Could you check a few things on this model? Use its own coordinates, in mm. A direction names the side the tool comes from. Give positions to 0.01 mm unless a question says otherwise; leave off trailing zeros. Write each loop counter-clockwise with the first axis right and the second up, starting at its lowest first coordinate (ties: lowest second). Pieces come first, ordered by that corner, then holes. Notation, with made-up numbers: M 55.5,35 L 105.5,35 A19 cw 105.5,48 Z; hole C 20.25,39.5 d3. An arc over 180 degrees is marked long. Use one line per item in the form item = value.
from build123d import *

# Parameters (mm, degrees)
F0_R     = 2
F0_R_2   = 6
F0_W     = 51.13
F0_H     = 19.04
F1_DEPTH = 25


# Not quite as in the source:
# - ends of sketch curves that miss each other by under 0.0002 mm in the source are joined


with BuildPart() as f1:
    # F0 (on Front) → F1 (new body)
    with BuildSketch(Plane.XZ):
        with BuildLine():
            Line((-0.0546134975, 0), (0, 0))
            Line((0, 0), (39.9453865025, 1.14717e-05))
            Line((39.9453865025, 1.14717e-05), (39.9453865025, 10.0000114717))
            Line((39.9453865025, 10.0000114717), (29.9453865025, 10.0000114717))
            Line((29.9453865025, 10.0000114717), (29.9576031817, 39.0801515195))
            ThreePointArc((29.9576031817, 39.0801515195), (24.9768942877, 34.5421678148), (20, 39.0843347471))
            ThreePointArc((20, 39.0843347471), (19.9842488656, 39.3130102593), (19.9789948068, 39.5421673735))
            ThreePointArc((19.9789948068, 39.5421673735), (14.7708428858, 35.0052540588), (10, 40))
            ThreePointArc((10, 40), (5, 35), (0, 40))
            ThreePointArc((0, 40), (-5, 35), (-10, 40))
            ThreePointArc((-10, 40), (-15, 35), (-20, 40))
            ThreePointArc((-20, 40), (-25, 35), (-30, 40))
            Line((-30, 40), (-30, 10))
            Line((-30, 10), (-40, 10))
            Line((-40, 10), (-40, 0))
            Line((-40, 0), (-0.0546134975, 0))
        make_face()
        with Locations((-35, 5)):
            Circle(F0_R, mode=Mode.SUBTRACT)
        with Locations((34.9453865025, 5.0000114717)):
            Circle(F0_R, mode=Mode.SUBTRACT)
        with BuildLine():
            ThreePointArc((20, 39.0843347471), (24.9768942877, 34.5421678148), (29.9576031817, 39.0801515195))
            Line((29.9576031817, 39.0801515195), (29.9579896136, 40))
            Line((29.9579896136, 40), (29.9747937682, 80))
            ThreePointArc((29.9747937682, 80), (24.9873968841, 75.3547848935), (20, 80))
            Line((20, 80), (20, 40))
            Line((20, 40), (20, 39.0843347471))
        make_face()
        with BuildLine():
            Line((29.9579896136, 40), (29.9576031817, 39.0801515195))
            ThreePointArc((29.9576031817, 39.0801515195), (29.9789943656, 39.5400668544), (29.9579896136, 40))
        make_face()
        with BuildLine():
            Line((-30, 80), (-30, 40))
            ThreePointArc((-30, 40), (-25, 35), (-20, 40))
            Line((-20, 40), (-20, 80))
            ThreePointArc((-20, 80), (-25, 75), (-30, 80))
        make_face()
        with BuildLine():
            Line((-30, 120), (-30, 80))
            ThreePointArc((-30, 80), (-25, 75), (-20, 80))
            Line((-20, 80), (-20, 120))
            ThreePointArc((-20, 120), (-25, 115), (-30, 120))
        make_face()
        with BuildLine():
            ThreePointArc((20, 80), (24.9873968841, 75.3547848935), (29.9747937682, 80))
            Line((29.9747937682, 80), (29.9915979227, 120))
            ThreePointArc((29.9915979227, 120), (24.9957989614, 115.2049212963), (20, 120))
            Line((20, 120), (20, 80))
        make_face()
        with BuildLine():
            Line((-30, 140), (-30, 120))
            ThreePointArc((-30, 120), (-25, 115), (-20, 120))
            Line((-20, 120), (-20, 140))
            Line((-20, 140), (-30, 140))
        make_face()
        with BuildLine():
            ThreePointArc((20, 120), (24.9957989614, 115.2049212963), (29.9915979227, 120))
            Line((29.9915979227, 120), (30, 140))
            Line((30, 140), (20, 140))
            Line((20, 140), (20, 120))
        make_face()
        Polygon((-40, 140), (-30, 140), (-20, 140), (-10, 140), (0, 140), (10, 140), (20, 140), (30, 140), (40, 140), (40, 220), (30, 220), (-30, 220), (-40, 220), align=None)
        with Locations((-35, 215)):
            Circle(F0_R, mode=Mode.SUBTRACT)
        with Locations((-20, 156)):
            Circle(F0_R_2, mode=Mode.SUBTRACT)
        with Locations((-15, 170)):
            Circle(F0_R, mode=Mode.SUBTRACT)
        with Locations((-5, 156)):
            Circle(F0_R, mode=Mode.SUBTRACT)
        with Locations((-5, 170)):
            Circle(F0_R, mode=Mode.SUBTRACT)
        with Locations((5, 170)):
            Circle(F0_R, mode=Mode.SUBTRACT)
        with Locations((15, 170)):
            Circle(F0_R, mode=Mode.SUBTRACT)
        with Locations((0, 189.52)):
            Rectangle(F0_W, F0_H, mode=Mode.SUBTRACT)
        with Locations((35, 215)):
            Circle(F0_R, mode=Mode.SUBTRACT)
        Polygon((-30, 230), (-30, 220), (30, 220), (30, 230), (0, 230), align=None)
        Polygon((-20, 250), (-30, 230), (0, 230), (30, 230), (20, 250), (0, 250), align=None)
        Polygon((0, 300), (-20, 250), (0, 250), (20, 250), align=None)
        with BuildLine():
            Line((-20, 120), (-20, 80))
            ThreePointArc((-20, 80), (-15, 75), (-10, 80))
            Line((-10, 80), (-10, 120))
            ThreePointArc((-10, 120), (-15, 115), (-20, 120))
        make_face()
        with BuildLine():
            Line((-10, 120), (-10, 80))
            ThreePointArc((-10, 80), (-5, 75), (0, 80))
            Line((0, 80), (0, 120))
            ThreePointArc((0, 120), (-5, 115), (-10, 120))
        make_face()
        with BuildLine():
            ThreePointArc((0, 80), (5, 75), (10, 80))
            Line((10, 80), (10, 120))
            ThreePointArc((10, 120), (5, 115), (0, 120))
            Line((0, 120), (0, 80))
        make_face()
        with BuildLine():
            ThreePointArc((10, 80), (15, 75), (20, 80))
            Line((20, 80), (20, 120))
            ThreePointArc((20, 120), (15, 115), (10, 120))
            Line((10, 120), (10, 80))
        make_face()
        with BuildLine():
            ThreePointArc((19.9789948068, 39.5421673735), (19.9842488656, 39.7713244878), (20, 40))
            Line((20, 40), (20, 80))
            ThreePointArc((20, 80), (15, 75), (10, 80))
            Line((10, 80), (10, 40))
            ThreePointArc((10, 40), (14.7708428858, 35.0052540588), (19.9789948068, 39.5421673735))
        make_face()
        with BuildLine():
            ThreePointArc((0, 40), (5, 35), (10, 40))
            Line((10, 40), (10, 80))
            ThreePointArc((10, 80), (5, 75), (0, 80))
            Line((0, 80), (0, 40))
        make_face()
        with BuildLine():
            Line((-10, 80), (-10, 40))
            ThreePointArc((-10, 40), (-5, 35), (0, 40))
            Line((0, 40), (0, 80))
            ThreePointArc((0, 80), (-5, 75), (-10, 80))
        make_face()
        with BuildLine():
            Line((-20, 80), (-20, 40))
            ThreePointArc((-20, 40), (-15, 35), (-10, 40))
            Line((-10, 40), (-10, 80))
            ThreePointArc((-10, 80), (-15, 75), (-20, 80))
        make_face()
        with BuildLine():
            Line((-20, 140), (-20, 120))
            ThreePointArc((-20, 120), (-15, 115), (-10, 120))
            Line((-10, 120), (-10, 140))
            Line((-10, 140), (-20, 140))
        make_face()
        with BuildLine():
            Line((-10, 140), (-10, 120))
            ThreePointArc((-10, 120), (-5, 115), (0, 120))
            Line((0, 120), (0, 140))
            Line((0, 140), (-10, 140))
        make_face()
        with BuildLine():
            ThreePointArc((0, 120), (5, 115), (10, 120))
            Line((10, 120), (10, 140))
            Line((10, 140), (0, 140))
            Line((0, 140), (0, 120))
        make_face()
        with BuildLine():
            ThreePointArc((10, 120), (15, 115), (20, 120))
            Line((20, 120), (20, 140))
            Line((20, 140), (10, 140))
            Line((10, 140), (10, 120))
        make_face()
    extrude(amount=F1_DEPTH)


solid = f1.part
1) If I drill on L1, parallel to Z at x = 35, y = -12.5; L2, parallel to X at y = -19.25, z = 170; L3, parallel to X at y = -18.75, z = 215, over which ranges is the centre line in solid material (lowest first)?
Checked values:
L1 = 0 to 3, 7 to 10, 140 to 213, 217 to 220
L2 = -40 to -17, -13 to -7, -3 to 3, 7 to 13, 17 to 40
L3 = -40 to -37, -33 to 33, 37 to 40
2) For faces 1 (the flat face through (-30, -12, 225)), 2 (the flat face through (-25.565, -12, 189)), 3 (the flat face through (-30, -12, 76)), 4 (the flat face through (35, -12, 10)), which set-ups out of +Z, -Z, +X, -X, +Y, -Y let a thin tool reach every point of the face, with its end or its side?
Checked values:
face_1 = +Z, -X, +Y, -Y
face_2 = +Y, -Y
face_3 = -X, +Y, -Y
face_4 = +X, +Y, -Y
3) I want a section at B-B, the plane y = -9.5. Count the separate pieces of the cut face and the enclosed holes in it, plus the area to 3 significant figures.
Checked values:
separate_pieces = 1
enclosed_holes = 12
area = 16,400 mm2
4) Thinking about a two-plate mould opening in X: for faces 5 (the flat face through (25.565, -12, 189)), 6 (the flat face through (0, -12, 199.04)), 7 (the flat face through (10, -12, 275)), 8 (the flat face through (35, -12, 140)), which applies, released by +X, released by -X, zero draft, split by the parting line, or undercut?
Checked values:
face_5 = undercut
face_6 = undercut
face_7 = released by +X
face_8 = zero draft
5) I want a section at D-D, the plane z = 55.5. Please give me the cut outline in (x, y), plus the area to 3 significant figures.
Checked values:
outline = M -30,-25 L 29.96,-25 L 29.96,0 L -30,0 Z
area = 1,500 mm2
6) I want a section at C-C, the plane z = 105. Please give me the cut outline in (x, y), plus the area to 3 significant figures.
Checked values:
outline = M -30,-25 L 29.99,-25 L 29.99,0 L -30,0 Z
area = 1,500 mm2
7) For pin 1 Ø8 at (y, z) = (-2.5, 112.5) entering from -X; pin 2 Ø3.5 at (x, z) = (-5, 156) entering from -Y; pin 3 Ø8 at (y, z) = (-20, 236) entering from +X; pin 4 Ø7.5 at (y, z) = (-17.5, 91) entering from +X, each with a flat end and sliding along its axis, tell me the tip position at first contact or that it passes through.
Checked values:
pin_1 = -30
pin_2 = through
pin_3 = 29
pin_4 = 29.98
8) I want a section at A-A, the plane z = 185. Please give me the cut outline in (x, y) (3 decimals), plus the area to 3 significant figures.
Checked values:
outline = M -40,-25 L -25.565,-25 L -25.565,0 L -40,0 Z; M 25.565,-25 L 40,-25 L 40,0 L 25.565,0 Z
area = 722 mm2
